Geometry check sheet. Reference: the model listing, model coordinates, mm. A direction names the side the tool comes from. Coordinates: 2 decimals unless noted, no trailing zeros. Loops run counter-clockwise (first coordinate to the right, second up) from the corner with the lowest first, then second, coordinate; pieces in that order, holes last.
from build123d import *

# Parameters (mm, degrees)
F1_DEPTH = 150
F2_W     = 24
F2_H     = 5.125
F3_DEPTH = 0.1
F4_DEPTH = 0.1


# Not quite as in the source:
# - ends of sketch curves that miss each other by under 0.0002 mm in the source are joined


with BuildPart() as f1:
    # F0 (on Front) → F1 (new body)
    with BuildSketch(Plane.XZ):
        with BuildLine():
            Line((53.992555, -15.220268), (57.083133, -14.095389))
            ThreePointArc((57.083133, -14.095389), (62.9018568836, -10.252747544), (66.3544503107, -4.1944440905))
            ThreePointArc((66.3544503107, -4.1944440905), (66.1141142416, -2.8747683688), (64.914288, -2.275))
            Line((64.914288, -2.275), (60.670593, -2.275))
            ThreePointArc((60.670593, -2.275), (59.8472095147, -2.5211899521), (59.2941043505, -3.1789471518))
            ThreePointArc((59.2941043505, -3.1789471518), (56.9827494729, -6.2209259886), (53.52425904, -7.8441451998))
            ThreePointArc((53.52425904, -7.8441451998), (52.6431740995, -8.0626756758), (51.7855370008, -8.3602070021))
            ThreePointArc((51.7855370008, -8.3602070021), (39.452831, 0), (51.7855371982, 8.3602074972))
            ThreePointArc((51.7855371982, 8.3602074972), (52.6431743712, 8.0626765952), (53.524259133, 7.844145664))
            ThreePointArc((53.524259133, 7.844145664), (56.9827494729, 6.2209259886), (59.2941043849, 3.1789471667))
            ThreePointArc((59.2941043849, 3.1789471667), (59.8472095147, 2.5211899521), (60.670593, 2.275))
            Line((60.670593, 2.275), (64.914288, 2.275))
            ThreePointArc((64.914288, 2.275), (66.1141145297, 2.8747687527), (66.3544497778, 4.1944449353))
            ThreePointArc((66.3544497778, 4.1944449353), (62.9018565554, 10.2527478944), (57.0831331177, 14.0953893235))
            Line((57.0831331177, 14.0953893235), (53.992555, 15.220268))
            ThreePointArc((53.992555, 15.220268), (52.3736165632, 15.715360306), (50.7118440801, 16.0387645685))
            Line((50.7118440801, 16.0387645685), (40.585713, 17.465))
            Line((40.585713, 17.465), (35.885713, 17.465))
            ThreePointArc((35.885713, 17.465), (35.6735809656, 17.5528679656), (35.585713, 17.765))
            Line((35.585713, 17.765), (35.585713, 18.7))
            ThreePointArc((35.585713, 18.7), (35.4978450344, 18.9121320344), (35.285713, 19))
            Line((35.285713, 19), (18.585713, 19))
            Line((18.585713, 19), (12.836393, 18.04178))
            ThreePointArc((12.836393, 18.04178), (12.656806899, 17.9397743434), (12.585713, 17.745862))
            Line((12.585713, 17.745862), (12.585713, 6.875))
            ThreePointArc((12.585713, 6.875), (12.6735809656, 6.6628679656), (12.885713, 6.575))
            Line((12.885713, 6.575), (18.285713, 6.575))
            ThreePointArc((18.285713, 6.575), (18.4978450344, 6.6628679656), (18.585713, 6.875))
            Line((18.585713, 6.875), (18.585713, 12.7))
            ThreePointArc((18.585713, 12.7), (18.6735809656, 12.9121320344), (18.885713, 13))
            Line((18.885713, 13), (26.285713, 13))
            ThreePointArc((26.285713, 13), (26.4978450344, 12.9121320344), (26.585713, 12.7))
            Line((26.585713, 12.7), (26.585713, 10.3))
            ThreePointArc((26.585713, 10.3), (26.6735809656, 10.0878679656), (26.885713, 10))
            Line((26.885713, 10), (32.285713, 10))
            ThreePointArc((32.285713, 10), (32.4978450344, 9.9121320344), (32.585713, 9.7))
            Line((32.585713, 9.7), (32.585713, -9.7))
            ThreePointArc((32.585713, -9.7), (32.4978450344, -9.9121320344), (32.285713, -10))
            Line((32.285713, -10), (26.885713, -10))
            ThreePointArc((26.885713, -10), (26.6735809656, -10.0878679656), (26.585713, -10.3))
            Line((26.585713, -10.3), (26.585713, -12.7))
            ThreePointArc((26.585713, -12.7), (26.4978450344, -12.9121320344), (26.285713, -13))
            Line((26.285713, -13), (18.885713, -13))
            ThreePointArc((18.885713, -13), (18.6735809656, -12.9121320344), (18.585713, -12.7))
            Line((18.585713, -12.7), (18.585713, -6.875))
            ThreePointArc((18.585713, -6.875), (18.4978450344, -6.6628679656), (18.285713, -6.575))
            Line((18.285713, -6.575), (12.885713, -6.575))
            ThreePointArc((12.885713, -6.575), (12.6735809656, -6.6628679656), (12.585713, -6.875))
            Line((12.585713, -6.875), (12.585713, -17.745862))
            ThreePointArc((12.585713, -17.745862), (12.656806899, -17.9397743434), (12.8363929795, -18.0417801231))
            Line((12.8363929795, -18.0417801231), (18.585713, -19))
            Line((18.585713, -19), (35.285713, -19))
            ThreePointArc((35.285713, -19), (35.4978450344, -18.9121320344), (35.585713, -18.7))
            Line((35.585713, -18.7), (35.585713, -17.765))
            ThreePointArc((35.585713, -17.765), (35.6735809656, -17.5528679656), (35.885713, -17.465))
            Line((35.885713, -17.465), (40.585713, -17.465))
            Line((40.585713, -17.465), (50.711844, -16.038764))
            ThreePointArc((50.711844, -16.038764), (52.3736165632, -15.715360306), (53.992555, -15.220268))
        make_face()
    extrude(amount=-F1_DEPTH)

    # F2 (on face) → F3 (join)
    with BuildSketch(Plane.YZ.offset(18.585713)):
        with Locations((37.5, 9.4375)):
            Rectangle(F2_W, F2_H)
    extrude(amount=F3_DEPTH)

    # F2 (on face) → F4 (join)
    with BuildSketch(Plane.YZ.offset(18.585713)):
        with Locations((37.5, -9.4375)):
            Rectangle(F2_W, F2_H)
    extrude(amount=F4_DEPTH)


solid = f1.part
(1) Gauge pin test, flat ends, axial feed: pin 1 Ø3 at (y, z) = (118, 5.5) entering from +X; pin 2 Ø4.5 at (x, y) = (63.5, 79) entering from +Z; pin 3 Ø5.5 at (y, z) = (38, -10.5) entering from +X. Record the tip position at first contact, or that the pin passes through.
Findings:
pin 1: stops at x = 66.4
pin 2: stops at z = 11.77
pin 3: stops at x = 64.8
(2) Sectioned sample at C-C on z = 0. Record the cut outline in (x, y), and give its area (3 significant figures).
Findings:
outline: (32.59, 0) - (39.45, 0) - (39.45, 150) - (32.59, 150) - close
area: 1,030 mm2
(3) Scan lines: L1, parallel to Z at x = 27.5, y = 8.5; L2, parallel to Z at x = 25, y = 15; L3, parallel to X at y = 43, z = 0. Record each from-to range of solid material in increasing order.
Findings:
L1: z = -19 to -10, 10 to 19
L2: z = -19 to -13, 13 to 19
L3: x = 32.59 to 39.45
(4) Sectioned sample at A-A on x = 24. Record the cut outline in (y, z), and give its area (3 significant figures).
Findings:
outline: (0, -19) - (150, -19) - (150, -13) - (0, -13) - close; (0, 13) - (150, 13) - (150, 19) - (0, 19) - close
area: 1,800 mm2
(5) Sectioned sample at B-B on x = 42. Record the cut outline in (y, z).
Findings:
outline: (0, -17.27) - (150, -17.27) - (150, -6.27) - (0, -6.27) - close; (0, 6.27) - (150, 6.27) - (150, 17.27) - (0, 17.27) - close
(6) Access from +Z, -Z, +X, -X, +Y, -Y to the whole of each face (thin tool, end or side, straight path). Record for faces 1 (the flat face through (16, 74, 6.575)), 2 (the flat face through (18.586, 74, 10)), 3 (the flat face through (12.586, 74, -12)), 4 (the flat face through (63, 74, 2.275)), 5 (the cylindrical face through (56.941, 73.95, 6.255)).
Findings:
face 1: -X, +Y, -Y
face 2: none
face 3: +Z, -Z, -X, +Y, -Y
face 4: +X, +Y, -Y
face 5: +Y, -Y
(7) Draft check along X on faces 6 (the flat face through (18.686, 37, -9)), 7 (the flat face through (39, 150, 0)), 8 (the flat face through (45.72, 73.95, 16.74)). Enter one of: +X half, -X half, draft (parallel to the pull), parting line (faces both ways), or undercut.
Findings:
face 6: undercut
face 7: draft
face 8: +X half
